Input: part model. Units: mm. Frame: model coordinates. Face numbers are marked on the shaded views. A direction names the side the tool comes from. Coordinates: 2 decimals unless noted, no trailing zeros. Order: outer loops, then holes, each group sorted by start corner. A loop starts at its lowest first (then second) coordinate and runs counter-clockwise, first axis right, second up. Notation, with made-up numbers: (42, 60.5) -> (61, 60.5) arc R18 cw to (61, 86.5) -> close; hole circle Ø11 at (49.25, 73). An arc over 180 degrees is marked (long way). Answer as CSV lines item,"result".
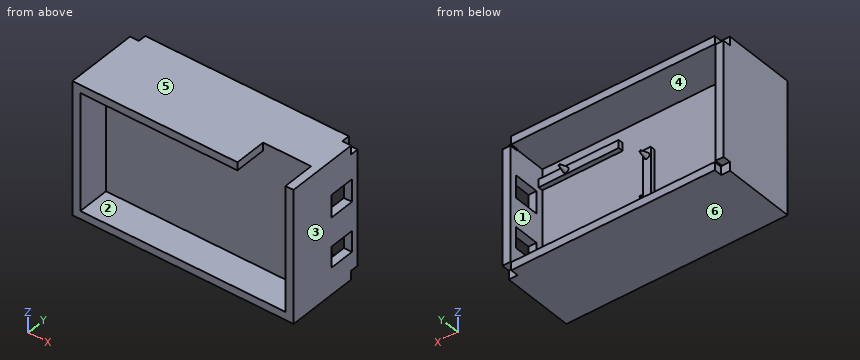
from build123d import *

# Parameters (mm, degrees)
SKETCH1_W                      = 138
SKETCH1_H                      = 83
BOSS_EXTRUDE1_DEPTH            = 5
SKETCH2_W                      = 138
SKETCH2_H                      = 83
SKETCH2_W_2                    = 128
SKETCH2_H_2                    = 73
BOSS_EXTRUDE2_DEPTH            = 20
CUT_EXTRUDE1_REACH             = 108.042
SKETCH3_W                      = 30
SKETCH3_H                      = 20
SKETCH4_W                      = 138
SKETCH4_H                      = 83
SKETCH4_W_2                    = 128
SKETCH4_H_2                    = 73
BOSS_EXTRUDE3_DEPTH            = 25
SKETCH5_W                      = 50
SKETCH5_H                      = 5
SKETCH5_W_2                    = 5
SKETCH5_H_2                    = 35
BOSS_EXTRUDE10_DEPTH           = 3
SKETCH6_R                      = 1.75
BOSS_EXTRUDE11_DEPTH           = 5
BOSS_EXTRUDE11_DRAFT           = 14
BOSS_EXTRUDE11_PROFILE_2_DEPTH = 5
BOSS_EXTRUDE11_PROFILE_2_DRAFT = 14
BOSS_EXTRUDE11_PROFILE_3_DEPTH = 5
BOSS_EXTRUDE11_PROFILE_3_DRAFT = 14
BOSS_EXTRUDE11_PROFILE_4_DEPTH = 5
BOSS_EXTRUDE11_PROFILE_4_DRAFT = 14
CUT_EXTRUDE2_REACH             = 144.518
SKETCH7_W                      = 13
SKETCH7_H                      = 16
CUT_EXTRUDE3_REACH             = 144.518
SKETCH8_W                      = 14
SKETCH8_H                      = 16
SKETCH11_W                     = 5.5
SKETCH11_H                     = 5.5
CUT_EXTRUDE7_DEPTH             = 5


with BuildPart() as part:
    # Sketch1 → Boss-Extrude1 (new body)
    with BuildSketch(Plane(origin=(0, 0, 0), x_dir=(1, 0, 0), z_dir=(0, 1, 0))):
        Rectangle(SKETCH1_W, SKETCH1_H)
    extrude(amount=BOSS_EXTRUDE1_DEPTH)

    # Sketch2 → Boss-Extrude2 (add)
    with BuildSketch(Plane.XZ):
        Rectangle(SKETCH2_W, SKETCH2_H)
        Rectangle(SKETCH2_W_2, SKETCH2_H_2, mode=Mode.SUBTRACT)
    extrude(amount=BOSS_EXTRUDE2_DEPTH)

    # Sketch3 → Cut-Extrude1 (cut, up to next)
    with BuildSketch(Plane(origin=(0, 0, 36.5), x_dir=(-1, 0, 0), z_dir=(0, 0, -1)), mode=Mode.PRIVATE) as cut_extrude1_sk1:
        with Locations((-49, -10)):
            Rectangle(SKETCH3_W, SKETCH3_H)
    cut_extrude1_tool1 = extrude(cut_extrude1_sk1.sketch, amount=-CUT_EXTRUDE1_REACH, mode=Mode.PRIVATE) & part.part
    add(cut_extrude1_tool1.solids().sort_by_distance((49, -10, 36.5))[0], mode=Mode.SUBTRACT)

    # Sketch4 → Boss-Extrude3 (add)
    with BuildSketch(Plane(origin=(0, 5, 0), x_dir=(1, 0, 0), z_dir=(0, 1, 0))):
        Rectangle(SKETCH4_W, SKETCH4_H)
        Rectangle(SKETCH4_W_2, SKETCH4_H_2, mode=Mode.SUBTRACT)
    extrude(amount=BOSS_EXTRUDE3_DEPTH)

    # Sketch5 → Boss-Extrude10 (add)
    with BuildSketch(Plane(origin=(0, 5, 0), x_dir=(1, 0, 0), z_dir=(0, 1, 0))):
        with Locations((39, -26)):
            Rectangle(SKETCH5_W, SKETCH5_H)
        with Locations((39, 23)):
            Rectangle(SKETCH5_W, SKETCH5_H)
        with Locations((-3.5, 3)):
            Rectangle(SKETCH5_W_2, SKETCH5_H_2)
    extrude(amount=BOSS_EXTRUDE10_DEPTH)


with BuildPart() as boss_extrude11_tool:
    # Sketch6 → Boss-Extrude11 (with draft: the straight prism first)
    with BuildSketch(Plane(origin=(0, 8, 0), x_dir=(1, 0, 0), z_dir=(0, 1, 0))):
        with Locations((47, 23)):
            Circle(SKETCH6_R)
    extrude(amount=BOSS_EXTRUDE11_DEPTH)
    # Boss-Extrude11: the draft: its side faces are tilted about the plane it starts from
    boss_extrude11_sides = [boss_extrude11_tool.faces().sort_by_distance(p)[0] for p in [
        (45.25, 10.5, -23),
    ]]
    draft(boss_extrude11_sides, Plane(origin=(0, 8, 0), x_dir=(1, 0, 0), z_dir=(0, 1, 0)), BOSS_EXTRUDE11_DRAFT)


with BuildPart() as part_1:
    add(part.part)

    # Boss-Extrude11: add boss_extrude11_tool
    add(boss_extrude11_tool.part)


with BuildPart() as boss_extrude11_profile_2_tool:
    # Sketch6 → Boss-Extrude11 profile 2 (with draft: the straight prism first)
    with BuildSketch(Plane(origin=(0, 8, 0), x_dir=(1, 0, 0), z_dir=(0, 1, 0))):
        with Locations((47, -26)):
            Circle(SKETCH6_R)
    extrude(amount=BOSS_EXTRUDE11_PROFILE_2_DEPTH)
    # Boss-Extrude11 profile 2: the draft: its side faces are tilted about the plane it starts from
    boss_extrude11_profile_2_sides = [boss_extrude11_profile_2_tool.faces().sort_by_distance(p)[0] for p in [
        (45.25, 10.5, 26),
    ]]
    draft(boss_extrude11_profile_2_sides, Plane(origin=(0, 8, 0), x_dir=(1, 0, 0), z_dir=(0, 1, 0)), BOSS_EXTRUDE11_PROFILE_2_DRAFT)


with BuildPart() as part_2:
    add(part_1.part)

    # Boss-Extrude11 profile 2: add boss_extrude11_profile_2_tool
    add(boss_extrude11_profile_2_tool.part)


with BuildPart() as boss_extrude11_profile_3_tool:
    # Sketch6 → Boss-Extrude11 profile 3 (with draft: the straight prism first)
    with BuildSketch(Plane(origin=(0, 8, 0), x_dir=(1, 0, 0), z_dir=(0, 1, 0))):
        with Locations((-3.5, 18)):
            Circle(SKETCH6_R)
    extrude(amount=BOSS_EXTRUDE11_PROFILE_3_DEPTH)
    # Boss-Extrude11 profile 3: the draft: its side faces are tilted about the plane it starts from
    boss_extrude11_profile_3_sides = [boss_extrude11_profile_3_tool.faces().sort_by_distance(p)[0] for p in [
        (-5.25, 10.5, -18),
    ]]
    draft(boss_extrude11_profile_3_sides, Plane(origin=(0, 8, 0), x_dir=(1, 0, 0), z_dir=(0, 1, 0)), BOSS_EXTRUDE11_PROFILE_3_DRAFT)


with BuildPart() as part_3:
    add(part_2.part)

    # Boss-Extrude11 profile 3: add boss_extrude11_profile_3_tool
    add(boss_extrude11_profile_3_tool.part)


with BuildPart() as boss_extrude11_profile_4_tool:
    # Sketch6 → Boss-Extrude11 profile 4 (with draft: the straight prism first)
    with BuildSketch(Plane(origin=(0, 8, 0), x_dir=(1, 0, 0), z_dir=(0, 1, 0))):
        with Locations((-3.5, -10)):
            Circle(SKETCH6_R)
    extrude(amount=BOSS_EXTRUDE11_PROFILE_4_DEPTH)
    # Boss-Extrude11 profile 4: the draft: its side faces are tilted about the plane it starts from
    boss_extrude11_profile_4_sides = [boss_extrude11_profile_4_tool.faces().sort_by_distance(p)[0] for p in [
        (-5.25, 10.5, 10),
    ]]
    draft(boss_extrude11_profile_4_sides, Plane(origin=(0, 8, 0), x_dir=(1, 0, 0), z_dir=(0, 1, 0)), BOSS_EXTRUDE11_PROFILE_4_DRAFT)


with BuildPart() as part_4:
    add(part_3.part)

    # Boss-Extrude11 profile 4: add boss_extrude11_profile_4_tool
    add(boss_extrude11_profile_4_tool.part)

    # Sketch7 → Cut-Extrude2 (cut, up to next)
    with BuildSketch(Plane.ZY.offset(-64), mode=Mode.PRIVATE) as cut_extrude2_sk1:
        with Locations((-18.25, 17.6)):
            Rectangle(SKETCH7_W, SKETCH7_H)
    cut_extrude2_tool1 = extrude(cut_extrude2_sk1.sketch, amount=-CUT_EXTRUDE2_REACH, mode=Mode.PRIVATE) & part_4.part
    add(cut_extrude2_tool1.solids().sort_by_distance((64, 17.6, -18.25))[0], mode=Mode.SUBTRACT)

    # Sketch8 → Cut-Extrude3 (cut, up to next)
    with BuildSketch(Plane.ZY.offset(-64), mode=Mode.PRIVATE) as cut_extrude3_sk1:
        with Locations((13.25, 17.6)):
            Rectangle(SKETCH8_W, SKETCH8_H)
    cut_extrude3_tool1 = extrude(cut_extrude3_sk1.sketch, amount=-CUT_EXTRUDE3_REACH, mode=Mode.PRIVATE) & part_4.part
    add(cut_extrude3_tool1.solids().sort_by_distance((64, 17.6, 13.25))[0], mode=Mode.SUBTRACT)

    # Sketch11 → Cut-Extrude7 (cut)
    with BuildSketch(Plane(origin=(0, 30, 0), x_dir=(1, 0, 0), z_dir=(0, 1, 0))):
        with Locations((-66.25, 38.75)):
            Rectangle(SKETCH11_W, SKETCH11_H)
        with Locations((-66.25, -38.75)):
            Rectangle(SKETCH11_W, SKETCH11_H)
        with Locations((66.25, -38.75)):
            Rectangle(SKETCH11_W, SKETCH11_H)
        with Locations((66.25, 38.75)):
            Rectangle(SKETCH11_W, SKETCH11_H)
    extrude(amount=-CUT_EXTRUDE7_DEPTH, mode=Mode.SUBTRACT)


solid = part_4.part
1. Cut plane B-B (y = 16.5). Return the cut outline in (x, z), plus the area to 4 significant figures.
Findings:
outline,"(-69, -41.5) -> (69, -41.5) -> (69, -24.75) -> (64, -24.75) -> (64, -36.5) -> (-64, -36.5) -> (-64, 36.5) -> (64, 36.5) -> (64, 20.25) -> (69, 20.25) -> (69, 41.5) -> (-69, 41.5) -> close; (64, -11.75) -> (69, -11.75) -> (69, 6.25) -> (64, 6.25) -> close"
area,"1,975 mm2"
2. Mould query, pull axis Z, two halves, no side actions, for the marked faces 4, 5 and 6. Classes: released by +Z, released by -Z, zero draft, split by the parting line, or undercut.
Findings:
face 4,"undercut"
face 5,"released by +Z"
face 6,"released by -Z"
3. Contact query for flat-ended pins moving along their axis: pin 1 (1.5 mm diameter, centred on x = -67.5, y = 26.5, fed in from +Z); pin 2 (1.6 mm diameter, centred on x = 66.5, z = -40, fed in from +Y); pin 3 (3 mm diameter, centred on x = -21.5, z = 5.5, fed in from -Y). Output: stop coordinate, or through.
Findings:
pin 1,"stops at z = 36"
pin 2,"stops at y = 25"
pin 3,"stops at y = 0"
4. Ray query, line 1 along Z through (x, y) = (25.5, 9); line 2 along X through (y, z) = (-7, 36); line 3 along X through (y, z) = (6, 28). Return the intervals inside material, ascending.
Findings:
line 1,"z = -41.5 to -36.5, 36.5 to 41.5"
line 2,"x = -69 to -64, 64 to 69"
line 3,"x = -69 to -64, 14 to 69"
5. Cut plane A-A (x = 10.5). Return the cut outline in (y, z).
Findings:
outline,"(-20, -41.5) -> (30, -41.5) -> (30, -36.5) -> (5, -36.5) -> (5, 36.5) -> (30, 36.5) -> (30, 41.5) -> (-20, 41.5) -> (-20, 36.5) -> (0, 36.5) -> (0, -36.5) -> (-20, -36.5) -> close"
6. Cut plane C-C (y = -3). Return the cut outline in (x, z).
Findings:
outline,"(-69, -41.5) -> (69, -41.5) -> (69, 41.5) -> (64, 41.5) -> (64, -36.5) -> (-64, -36.5) -> (-64, 36.5) -> (34, 36.5) -> (34, 41.5) -> (-69, 41.5) -> close"
7. Reachability of the marked faces 1, 2 and 3 from +Z, -Z, +X, -X, +Y, -Y: full face, straight path, thin tool, end or side. Return the list, or none.
Findings:
face 1,"+Y"
face 2,"-Y"
face 3,"+Z, -Z, +X, +Y, -Y"
8. Cut plane D-D (x = 41.5). Return the cut outline in (y, z).
Findings:
outline,"(-20, -41.5) -> (30, -41.5) -> (30, -36.5) -> (5, -36.5) -> (5, -25.5) -> (8, -25.5) -> (8, -20.5) -> (5, -20.5) -> (5, 23.5) -> (8, 23.5) -> (8, 28.5) -> (5, 28.5) -> (5, 36.5) -> (30, 36.5) -> (30, 41.5) -> (0, 41.5) -> (0, -36.5) -> (-20, -36.5) -> close"
